Can you work these out from the model? Positions are in its coordinate system, mm. A direction names the side the tool comes from. Round coordinates to 2 decimals unless told otherwise and drop trailing zeros. Write each loop counter-clockwise with the first axis right and the second up, starting at its lowest first coordinate (ties: lowest second). Pieces come first, ordered by that corner, then holes.
Q1. If we section it at B-B (z = 0): Please give me the cut outline in (x, y).
Q2. Please list where these lines run through material, in increasing order: line 1 along Z through (x, y) = (-13.5, 11) (3 decimals); line 2 along X through (y, z) = (37.5, -5.5); line 3 along Y through (x, z) = (35, 4).
Q3. If we section it at C-C (y = 26.5): Give the number of separate pieces and of enclosed holes in the cut face, plus the area to 3 significant figures.
Q4. I'm going to push flat-ended pins straight in: pin 1 Ø2 at (y, z) = (7, -17) entering from +X; pin 2 Ø6 at (y, z) = (13, -16) entering from -X; pin 3 Ø2.5 at (y, z) = (40, -7.5) entering from +X; pin 4 Ø5 at (x, z) = (-33.5, 0) entering from +Y. Where does each tip first touch, or does it pass through?
Q5. We'd pull the mould along Z, two halves only. Please class faces 5 (the flat face through (0, 40, -11.049)), 6 (the flat face through (16.224, 26, 7)), 7 (the flat face through (-20.574, 40, 0)), 8 (the flat face through (36.1, 14.4, 13)): +Z half, -Z half, draft (parallel to the pull), parting line (faces both ways), or undercut.
Q6. If we section it at A-A (x = -8.5): Please give me the cut outline in (y, z) (3 decimals), plus the area to 3 significant figures.
Q7. For faces 1 (the flat face through (18, 26, 4.159)), 2 (the flat face through (17.018, 40, -7)), 3 (the flat face through (-17.018, 40, -7)), 4 (the flat face through (20.574, 40, 0)), which set-ups out of +Z, -Z, +X, -X, +Y, -Y let a thin tool reach every point of the face, with its end or its side?
Q8. If we section it at D-D (x = 32): Please give me the cut outline in (y, z).
from build123d import *

# Parameters (mm, degrees)
SKETCH1_R           = 3.175
BOSS_EXTRUDE1_DEPTH = 29.21
BOSS_EXTRUDE2_DEPTH = 22.86
CUT_EXTRUDE1_REACH  = 54.07


with BuildPart() as part:
    # Sketch1 → Boss-Extrude1 (new body)
    with BuildSketch(Plane(origin=(0, 0, 0), x_dir=(1, 0, 0), z_dir=(0, 1, 0))):
        with BuildLine():
            Line((30.607538026, 19.8480292), (41.428260842, 6.35684672))
            ThreePointArc((41.428260842, 6.35684672), (43.6626, 0), (41.428260842, -6.35684672))
            Line((41.428260842, -6.35684672), (30.607538026, -19.8480292))
            ThreePointArc((30.607538026, -19.8480292), (28.401158949, -21.599999363), (25.654, -22.225))
            Line((25.654, -22.225), (-25.654, -22.225))
            ThreePointArc((-25.654, -22.225), (-28.401158949, -21.599999363), (-30.607538026, -19.8480292))
            Line((-30.607538026, -19.8480292), (-41.428260842, -6.35684672))
            ThreePointArc((-41.428260842, -6.35684672), (-43.6626, 0), (-41.428260842, 6.35684672))
            Line((-41.428260842, 6.35684672), (-30.607538026, 19.8480292))
            ThreePointArc((-30.607538026, 19.8480292), (-28.401158949, 21.599999363), (-25.654, 22.225))
            Line((-25.654, 22.225), (25.654, 22.225))
            ThreePointArc((25.654, 22.225), (28.401158949, 21.599999363), (30.607538026, 19.8480292))
        make_face()
        with Locations((-33.5026, 0)):
            Circle(SKETCH1_R, mode=Mode.SUBTRACT)
        with Locations((33.5026, 0)):
            Circle(SKETCH1_R, mode=Mode.SUBTRACT)
    extrude(amount=BOSS_EXTRUDE1_DEPTH)

    # Sketch2 → Boss-Extrude2 (add)
    with BuildSketch(Plane(origin=(0, 29.21, 0), x_dir=(1, 0, 0), z_dir=(0, 1, 0))):
        with BuildLine():
            Line((-19.304, -4.953), (-17.018, -4.953))
            Line((-17.018, -4.953), (-17.018, 4.953))
            Line((-17.018, 4.953), (-19.304, 4.953))
            ThreePointArc((-19.304, 4.953), (-20.202025612, 4.581025612), (-20.574, 3.683))
            Line((-20.574, 3.683), (-20.574, -3.683))
            ThreePointArc((-20.574, -3.683), (-20.202025612, -4.581025612), (-19.304, -4.953))
        make_face()
        with BuildLine():
            ThreePointArc((-17.018, 9.779), (-16.646025612, 10.677025612), (-15.748, 11.049))
            Line((-15.748, 11.049), (15.748, 11.049))
            ThreePointArc((15.748, 11.049), (16.646025612, 10.677025612), (17.018, 9.779))
            Line((17.018, 9.779), (17.018, -9.779))
            ThreePointArc((17.018, -9.779), (16.646025612, -10.677025612), (15.748, -11.049))
            Line((15.748, -11.049), (-15.748, -11.049))
            ThreePointArc((-15.748, -11.049), (-16.646025612, -10.677025612), (-17.018, -9.779))
            Line((-17.018, -9.779), (-17.018, 9.779))
        make_face()
        with BuildLine():
            Line((17.018, 4.953), (17.018, -4.953))
            Line((17.018, -4.953), (19.304, -4.953))
            ThreePointArc((19.304, -4.953), (20.202025612, -4.581025612), (20.574, -3.683))
            Line((20.574, -3.683), (20.574, 3.683))
            ThreePointArc((20.574, 3.683), (20.202025612, 4.581025612), (19.304, 4.953))
            Line((19.304, 4.953), (17.018, 4.953))
        make_face()
    extrude(amount=BOSS_EXTRUDE2_DEPTH)

    # Sketch4 → Cut-Extrude1 (cut, up to next)
    with BuildSketch(Plane(origin=(0, 52.07, 0), x_dir=(1, 0, 0), z_dir=(0, 1, 0)), mode=Mode.PRIVATE) as cut_extrude1_sk1:
        with BuildLine():
            Line((-16.22425, 4.15925), (-16.22425, 9.779))
            ThreePointArc((-16.22425, 9.779), (-16.084759605, 10.115759605), (-15.748, 10.25525))
            Line((-15.748, 10.25525), (15.748, 10.25525))
            ThreePointArc((15.748, 10.25525), (16.084759605, 10.115759605), (16.22425, 9.779))
            Line((16.22425, 9.779), (16.22425, 4.15925))
            Line((16.22425, 4.15925), (19.304, 4.15925))
            ThreePointArc((19.304, 4.15925), (19.640759605, 4.019759605), (19.78025, 3.683))
            Line((19.78025, 3.683), (19.78025, -3.683))
            ThreePointArc((19.78025, -3.683), (19.640759605, -4.019759605), (19.304, -4.15925))
            Line((19.304, -4.15925), (16.22425, -4.15925))
            Line((16.22425, -4.15925), (16.22425, -9.779))
            ThreePointArc((16.22425, -9.779), (16.084759605, -10.115759605), (15.748, -10.25525))
            Line((15.748, -10.25525), (-15.748, -10.25525))
            ThreePointArc((-15.748, -10.25525), (-16.084759605, -10.115759605), (-16.22425, -9.779))
            Line((-16.22425, -9.779), (-16.22425, -4.15925))
            Line((-16.22425, -4.15925), (-19.304, -4.15925))
            ThreePointArc((-19.304, -4.15925), (-19.640759605, -4.019759605), (-19.78025, -3.683))
            Line((-19.78025, -3.683), (-19.78025, 3.683))
            ThreePointArc((-19.78025, 3.683), (-19.640759605, 4.019759605), (-19.304, 4.15925))
            Line((-19.304, 4.15925), (-16.22425, 4.15925))
        make_face()
    cut_extrude1_tool1 = extrude(cut_extrude1_sk1.sketch, amount=-CUT_EXTRUDE1_REACH, mode=Mode.PRIVATE) & part.part
    add(cut_extrude1_tool1.solids().sort_by_distance((0, 52.07, 0))[0], mode=Mode.SUBTRACT)


solid = part.part
A:
1. outline: (-43.66, 0) - (-36.68, 0) - (-36.68, 29.21) - (-43.66, 29.21) - close; (-30.33, 0) - (-19.78, 0) - (-19.78, 52.07) - (-20.57, 52.07) - (-20.57, 29.21) - (-30.33, 29.21) - close; (19.78, 0) - (30.33, 0) - (30.33, 29.21) - (20.57, 29.21) - (20.57, 52.07) - (19.78, 52.07) - close; (36.68, 0) - (43.66, 0) - (43.66, 29.21) - (36.68, 29.21) - close
2. line 1: z = -22.225 to -10.255, 10.255 to 22.225
2. line 2: x = -17.02 to -16.22, 16.22 to 17.02
2. line 3: y = 0 to 29.21
3. separate pieces: 1
3. enclosed holes: 3
3. area: 2,520 mm2
4. pin 1: stops at x = 33.69
4. pin 2: stops at x = -36.1
4. pin 3: stops at x = 17.02
4. pin 4: passes through
5. face 5: -Z half
5. face 6: undercut
5. face 7: draft
5. face 8: +Z half
6. outline: (0, -22.225) - (29.21, -22.225) - (29.21, -11.049) - (52.07, -11.049) - (52.07, -10.255) - (0, -10.255) - close; (0, 10.255) - (52.07, 10.255) - (52.07, 11.049) - (29.21, 11.049) - (29.21, 22.225) - (0, 22.225) - close
6. area: 736 mm2
7. face 1: +Y, -Y
7. face 2: -Z, +X, +Y
7. face 3: -Z, -X, +Y
7. face 4: +Z, -Z, +X, +Y
8. outline: (0, -18.11) - (29.21, -18.11) - (29.21, -2.8) - (0, -2.8) - close; (0, 2.8) - (29.21, 2.8) - (29.21, 18.11) - (0, 18.11) - close
